from build123d import *

# Parameters (mm, degrees)
BOSS_EXTRUDE1_DEPTH = 3
CUT_EXTRUDE1_DEPTH  = 3
CUT_EXTRUDE3_START  = -117
CUT_EXTRUDE3_DEPTH  = 187
CUT_EXTRUDE5_DEPTH  = 3
CUT_EXTRUDE6_START  = -187
CUT_EXTRUDE6_DEPTH  = 3


with BuildPart() as part:
    # Sketch1 → Boss-Extrude1 (new body)
    with BuildSketch(Plane.XY):
        Polygon((10, 0), (190, 0), (190, 120), (9.862497021, 120), (0, 120), (0, 0), align=None)
    extrude(amount=BOSS_EXTRUDE1_DEPTH)

    # Sketch3 → Cut-Extrude1 (cut)
    with BuildSketch(Plane(origin=(0, 120, 0), x_dir=(1, 0, 0), z_dir=(0, 1, 0))):
        Polygon((181.0916961, -3), (182.183607, 0), (175.183607, 0), (176.275517, -3), align=None)
        Polygon((169.2716961, -3), (170.363607, 0), (163.363607, 0), (164.455517, -3), align=None)
        Polygon((157.4516961, -3), (158.543607, 0), (151.543607, 0), (152.635517, -3), align=None)
        Polygon((145.6316961, -3), (146.723607, 0), (139.723607, 0), (140.815517, -3), align=None)
        Polygon((133.8116961, -3), (134.903607, 0), (127.903607, 0), (128.995517, -3), align=None)
        Polygon((121.9916961, -3), (123.083607, 0), (116.083607, 0), (117.175517, -3), align=None)
        Polygon((110.1716961, -3), (111.263607, 0), (104.263607, 0), (105.355517, -3), align=None)
        Polygon((98.3516961, -3), (99.443607, 0), (92.443607, 0), (93.535517, -3), align=None)
        Polygon((86.5316961, -3), (87.623607, 0), (80.623607, 0), (81.715517, -3), align=None)
        Polygon((74.7116961, -3), (75.803607, 0), (68.803607, 0), (69.895517, -3), align=None)
        Polygon((62.8916961, -3), (63.983607, 0), (56.983607, 0), (58.075517, -3), align=None)
        Polygon((51.0716961, -3), (52.163607, 0), (45.163607, 0), (46.255517, -3), align=None)
        Polygon((39.2516961, -3), (40.343607, 0), (33.343607, 0), (34.435517, -3), align=None)
        Polygon((27.4316961, -3), (28.523607, 0), (21.523607, 0), (22.615517, -3), align=None)
        Polygon((15.6116961, -3), (16.703607, 0), (9.703607, 0), (10.795517, -3), align=None)
        Polygon((232.620596447, -14.855202406), (233.712507347, -11.855202406), (226.712507347, -11.855202406), (227.804417347, -14.855202406), align=None)
    extrude(amount=-CUT_EXTRUDE1_DEPTH, mode=Mode.SUBTRACT)

    # Sketch3<2> → Cut-Extrude3 (cut)
    with BuildSketch(Plane(origin=(0, 120, 0), x_dir=(1, 0, 0), z_dir=(0, 1, 0)).offset(CUT_EXTRUDE3_START)):
        Polygon((181.0916961, -3), (182.183607, 0), (175.183607, 0), (176.275517, -3), align=None)
        Polygon((169.2716961, -3), (170.363607, 0), (163.363607, 0), (164.455517, -3), align=None)
        Polygon((157.4516961, -3), (158.543607, 0), (151.543607, 0), (152.635517, -3), align=None)
        Polygon((145.6316961, -3), (146.723607, 0), (139.723607, 0), (140.815517, -3), align=None)
        Polygon((133.8116961, -3), (134.903607, 0), (127.903607, 0), (128.995517, -3), align=None)
        Polygon((121.9916961, -3), (123.083607, 0), (116.083607, 0), (117.175517, -3), align=None)
        Polygon((110.1716961, -3), (111.263607, 0), (104.263607, 0), (105.355517, -3), align=None)
        Polygon((98.3516961, -3), (99.443607, 0), (92.443607, 0), (93.535517, -3), align=None)
        Polygon((86.5316961, -3), (87.623607, 0), (80.623607, 0), (81.715517, -3), align=None)
        Polygon((74.7116961, -3), (75.803607, 0), (68.803607, 0), (69.895517, -3), align=None)
        Polygon((62.8916961, -3), (63.983607, 0), (56.983607, 0), (58.075517, -3), align=None)
        Polygon((51.0716961, -3), (52.163607, 0), (45.163607, 0), (46.255517, -3), align=None)
        Polygon((39.2516961, -3), (40.343607, 0), (33.343607, 0), (34.435517, -3), align=None)
        Polygon((27.4316961, -3), (28.523607, 0), (21.523607, 0), (22.615517, -3), align=None)
        Polygon((15.6116961, -3), (16.703607, 0), (9.703607, 0), (10.795517, -3), align=None)
        Polygon((232.620596447, -14.855202406), (233.712507347, -11.855202406), (226.712507347, -11.855202406), (227.804417347, -14.855202406), align=None)
    extrude(amount=-CUT_EXTRUDE3_DEPTH, mode=Mode.SUBTRACT)

    # Sketch6 → Cut-Extrude5 (cut)
    with BuildSketch(Plane.ZY):
        Polygon((0, 104.7919109), (3, 103.7), (3, 110.7), (0, 109.60809), align=None)
        Polygon((0, 92.9919109), (3, 91.9), (3, 98.9), (0, 97.80809), align=None)
        Polygon((0, 81.1919109), (3, 80.1), (3, 87.1), (0, 86.00809), align=None)
        Polygon((0, 69.3919109), (3, 68.3), (3, 75.3), (0, 74.20809), align=None)
        Polygon((0, 57.5919109), (3, 56.5), (3, 63.5), (0, 62.40809), align=None)
        Polygon((0, 45.7919109), (3, 44.7), (3, 51.7), (0, 50.60809), align=None)
        Polygon((0, 33.9919109), (3, 32.9), (3, 39.9), (0, 38.80809), align=None)
        Polygon((0, 22.1919109), (3, 21.1), (3, 28.1), (0, 27.00809), align=None)
        Polygon((0, 10.3919109), (3, 9.3), (3, 16.3), (0, 15.20809), align=None)
    extrude(amount=-CUT_EXTRUDE5_DEPTH, mode=Mode.SUBTRACT)

    # Sketch6<3> → Cut-Extrude6 (cut)
    with BuildSketch(Plane.ZY.offset(CUT_EXTRUDE6_START)):
        Polygon((0, 104.7919109), (3, 103.7), (3, 110.7), (0, 109.60809), align=None)
        Polygon((0, 92.9919109), (3, 91.9), (3, 98.9), (0, 97.80809), align=None)
        Polygon((0, 81.1919109), (3, 80.1), (3, 87.1), (0, 86.00809), align=None)
        Polygon((0, 69.3919109), (3, 68.3), (3, 75.3), (0, 74.20809), align=None)
        Polygon((0, 57.5919109), (3, 56.5), (3, 63.5), (0, 62.40809), align=None)
        Polygon((0, 45.7919109), (3, 44.7), (3, 51.7), (0, 50.60809), align=None)
        Polygon((0, 33.9919109), (3, 32.9), (3, 39.9), (0, 38.80809), align=None)
        Polygon((0, 22.1919109), (3, 21.1), (3, 28.1), (0, 27.00809), align=None)
        Polygon((0, 10.3919109), (3, 9.3), (3, 16.3), (0, 15.20809), align=None)
    extrude(amount=-CUT_EXTRUDE6_DEPTH, mode=Mode.SUBTRACT)


solid = part.part
Geometry check sheet. Reference: the model listing, model coordinates, mm. Give positions to 0.01 mm unless a question says otherwise; leave off trailing zeros. Write each loop counter-clockwise with the first axis right and the second up, starting at its lowest first coordinate (ties: lowest second). Pieces come first, ordered by that corner, then holes.
1) Thickness scan on line 1 (X direction, y = 74, z = 0.25); line 2 (Y direction, x = 58, z = 2.2). Record the ranges inside material, lowest first.
Values follow:
line 1: x = 3 to 187
line 2: y = 3 to 117
2) Cross-section at A-A (y = 95.5). Record the boundary of the cut face in (x, z).
Values follow:
outline: (3, 0) - (187, 0) - (187, 3) - (3, 3) - close
3) Cross-section at B-B (x = 155). Record the boundary of the cut face in (y, z), plus the area to 3 significant figures.
Values follow:
outline: (3, 0) - (117, 0) - (117, 3) - (3, 3) - close
area: 342 mm2
4) Go/stop test with flat-tipped pins: pin 1 Ø12 at (x, y) = (87, 103) entering from -Z; pin 2 Ø1.5 at (x, z) = (168, 1.5) entering from -Y; pin 3 Ø1.5 at (y, z) = (14.5, 1.5) entering from +X; pin 4 Ø0.9 at (x, z) = (37, 1) entering from +Y. Record where each tip stops, or that it passes through.
Values follow:
pin 1: stops at z = 0
pin 2: stops at y = 3
pin 3: stops at x = 187
pin 4: stops at y = 117
